The model under review builds one solid part; all positions refer to its coordinate system, in mm. Face numbers are marked on the shaded views. A direction names the side the tool comes from. Coordinates: 2 decimals unless noted, no trailing zeros. Order: outer loops, then holes, each group sorted by start corner. A loop starts at its lowest first (then second) coordinate and runs counter-clockwise, first axis right, second up. Notation, with made-up numbers: M 9.25,-2.75 L 63.25,-2.75 A23 cw 63.25,25.25 Z; hole C 83.25,83 d7. An arc over 180 degrees is marked long. One line per item, written item: value.
```python
from build123d import *

# Parameters (mm, degrees)
SKETCH_1_W          = 31
SKETCH_1_H          = 20
EXTRUDE_1_DEPTH     = 10.8
SKETCH_2_R          = 1.55
CUT_EXTRUDE_1_DEPTH = 22.37498538
FILLET_1_R          = 3
FILLET_2_R          = 3
SKETCH_3_W          = 15
SKETCH_3_H          = 5
CUT_EXTRUDE_2_DEPTH = 3


with BuildPart() as part:
    # 草图1 → 凸台-拉伸1 (new body)
    with BuildSketch(Plane.XY):
        Rectangle(SKETCH_1_W, SKETCH_1_H)
    extrude(amount=EXTRUDE_1_DEPTH)

    # 草图2 → 切除-拉伸1 (cut, through all)
    with BuildSketch(Plane(origin=(0, 0, 0), x_dir=(-1, 0, 0), z_dir=(0, 0, -1))):
        with Locations((-12.7, -7)):
            Circle(SKETCH_2_R)
        with Locations((12.7, -7)):
            Circle(SKETCH_2_R)
    extrude(amount=-CUT_EXTRUDE_1_DEPTH, mode=Mode.SUBTRACT)

    # 圆角1
    fillet_1_edges = [part.edges().sort_by_distance(p)[0] for p in [
        (-15.5, -10, 5.4),
    ]]
    fillet(fillet_1_edges, radius=FILLET_1_R)

    # 圆角2
    fillet_2_edges = [part.edges().sort_by_distance(p)[0] for p in [
        (15.5, -10, 5.4),
    ]]
    fillet(fillet_2_edges, radius=FILLET_2_R)

    # 草图3 → 切除-拉伸2 (cut)
    with BuildSketch(Plane.XZ.offset(10)):
        with Locations((0, 5.4)):
            Rectangle(SKETCH_3_W, SKETCH_3_H)
    extrude(amount=-CUT_EXTRUDE_2_DEPTH, mode=Mode.SUBTRACT)


solid = part.part
```
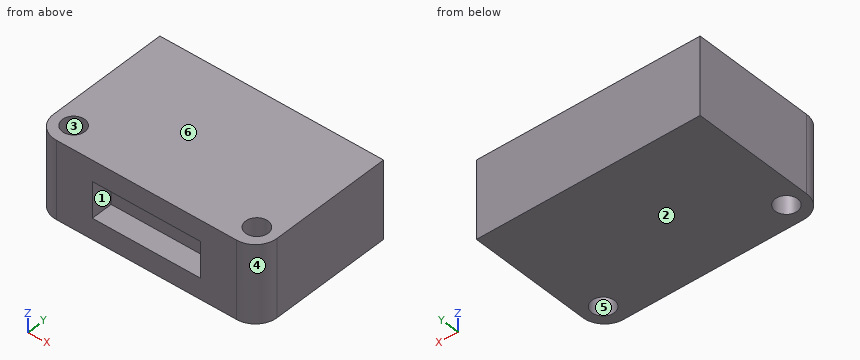
(1) We need section C-C, the plane x = 3. State the section outline as (y, z) points, plus the area to 3 significant figures.
Geometry results:
outline: M -10,0 L 10,0 L 10,10.8 L -10,10.8 L -10,7.9 L -7,7.9 L -7,2.9 L -10,2.9 Z
area: 201 mm2
(2) Mouldability with a two-part tool opening along Y and no side actions: class the marked faces 3, 4, 5 and 6 as +Y half, -Y half, draft (parallel to the pull), parting line (faces both ways), or undercut.
Geometry results:
face 3: undercut
face 4: -Y half
face 5: undercut
face 6: draft
(3) Insertion check: pin 1 Ø1.5 at (x, z) = (1, 5) entering from -Y; pin 2 Ø3.5 at (y, z) = (-9, 6) entering from +X; pin 3 Ø3 at (x, y) = (12.7, -7) entering from +Z (3 decimals). Each pin has a flat end and moves straight along its axis. Give the tip position at first contact, or say it passes through.
Geometry results:
pin 1: stops at y = -7
pin 2: stops at x = 15.49
pin 3: passes through
(4) For L1, parallel to Y at x = -12.7, z = 3; L2, parallel to X at y = -7.25, z = 8.5; L3, parallel to X at y = -8.25, z = 8.25, list the stretches that pass through material, from the lowest coordinate up.
Geometry results:
L1: y = -9.99 to -8.55, -5.45 to 10
L2: x = -15.49 to -14.23, -11.17 to 11.17, 14.23 to 15.49
L3: x = -15.23 to -13.62, -11.78 to 11.78, 13.62 to 15.23
(5) We need section A-A, the plane z = 4.75. State the section outline as (x, y) points.
Geometry results:
outline: M -15.5,-7 A3 ccw -12.5,-10 L -7.5,-10 L -7.5,-7 L 7.5,-7 L 7.5,-10 L 12.5,-10 A3 ccw 15.5,-7 L 15.5,10 L -15.5,10 Z; hole C -12.7,-7 d3.1; hole C 12.7,-7 d3.1
(6) We need section D-D, the plane z = 9. State the section outline as (x, y) points.
Geometry results:
outline: M -15.5,-7 A3 ccw -12.5,-10 L 12.5,-10 A3 ccw 15.5,-7 L 15.5,10 L -15.5,10 Z; hole C -12.7,-7 d3.1; hole C 12.7,-7 d3.1
(7) We need section B-B, the plane y = -7.75. State the section outline as (x, z) points, plus the area to 3 significant figures.
Geometry results:
outline: M -15.4,0 L -14.06,0 L -14.06,10.8 L -15.4,10.8 Z; M -11.34,0 L 11.34,0 L 11.34,10.8 L -11.34,10.8 Z; M 14.06,0 L 15.4,0 L 15.4,10.8 L 14.06,10.8 Z; hole M -7.5,2.9 L 7.5,2.9 L 7.5,7.9 L -7.5,7.9 Z
area: 199 mm2
(8) Tool access review of the marked faces 1 and 2: name each direction out of +Z, -Z, +X, -X, +Y, -Y from which nothing blocks a thin tool from reaching the whole face with its end or side.
Geometry results:
face 1: -Y
face 2: -Z, +X, -X, +Y, -Y
